CAD build for the part. Positions are in the model's coordinates, mm. Face numbers are marked on the shaded views. A direction names the side the tool comes from. Coordinates: 2 decimals unless noted, no trailing zeros. Loops run counter-clockwise (first coordinate to the right, second up) from the corner with the lowest first, then second, coordinate; pieces in that order, holes last. Notation, with made-up numbers: (71, -34) - (123, -34) arc R25 ccw to (123, -2) - close; hole circle Ø2 at (5, -11). An arc over 180 degrees is marked (long way). Put each result on its own line as item: value.
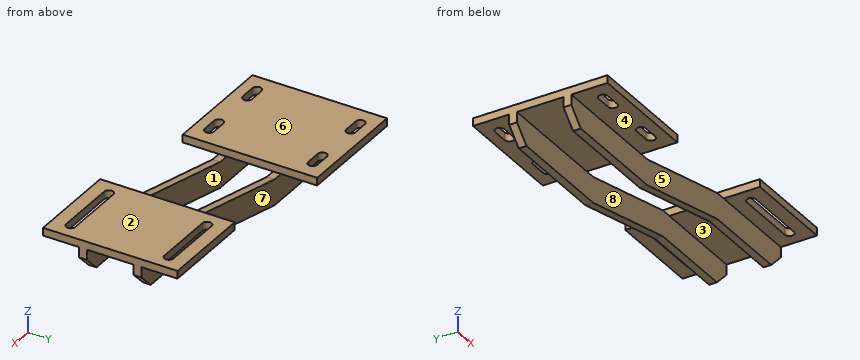
```python
from build123d import *

# Parameters (mm, degrees)
F0_W     = 139.7
F0_H     = 165.1
F1_DEPTH = 9.525
F3_W     = 114.3
F3_H     = 165.1
F4_DEPTH = 9.525
F7_DEPTH = 9.525
F9_SIZE  = 19.05


with BuildPart() as f1:
    # F0 (on Top) → F1 (new body)
    with BuildSketch(Plane.XY):
        Rectangle(F0_W, F0_H)
        with BuildLine():
            ThreePointArc((-47.625, -69.088), (-53.213, -63.5), (-47.625, -57.912))
            Line((-47.625, -57.912), (-28.575, -57.912))
            ThreePointArc((-28.575, -57.912), (-22.987, -63.5), (-28.575, -69.088))
            Line((-28.575, -69.088), (-47.625, -69.088))
        make_face(mode=Mode.SUBTRACT)
        with BuildLine():
            Line((28.575, -57.912), (47.625, -57.912))
            ThreePointArc((47.625, -57.912), (53.213, -63.5), (47.625, -69.088))
            Line((47.625, -69.088), (28.575, -69.088))
            ThreePointArc((28.575, -69.088), (22.987, -63.5), (28.575, -57.912))
        make_face(mode=Mode.SUBTRACT)
        with BuildLine():
            Line((-28.575, 57.912), (-47.625, 57.912))
            ThreePointArc((-47.625, 57.912), (-53.213, 63.5), (-47.625, 69.088))
            Line((-47.625, 69.088), (-28.575, 69.088))
            ThreePointArc((-28.575, 69.088), (-22.987, 63.5), (-28.575, 57.912))
        make_face(mode=Mode.SUBTRACT)
        with BuildLine():
            ThreePointArc((47.625, 69.088), (53.213, 63.5), (47.625, 57.912))
            Line((47.625, 57.912), (28.575, 57.912))
            ThreePointArc((28.575, 57.912), (22.987, 63.5), (28.575, 69.088))
            Line((28.575, 69.088), (47.625, 69.088))
        make_face(mode=Mode.SUBTRACT)
    extrude(amount=-F1_DEPTH)



with BuildPart() as f4:
    # F3 (on offset) → F4 (new body)
    with BuildSketch(Plane.XY.offset(31.75)):
        with Locations((292.1, 0)):
            Rectangle(F3_W, F3_H)
        with BuildLine():
            ThreePointArc((254, -65.913), (248.412, -60.325), (254, -54.737))
            Line((254, -54.737), (330.2, -54.737))
            ThreePointArc((330.2, -54.737), (335.788, -60.325), (330.2, -65.913))
            Line((330.2, -65.913), (254, -65.913))
        make_face(mode=Mode.SUBTRACT)
        with BuildLine():
            Line((330.2, 54.737), (254, 54.737))
            ThreePointArc((254, 54.737), (248.412, 60.325), (254, 65.913))
            Line((254, 65.913), (330.2, 65.913))
            ThreePointArc((330.2, 65.913), (335.788, 60.325), (330.2, 54.737))
        make_face(mode=Mode.SUBTRACT)
    extrude(amount=-F4_DEPTH)


with BuildPart() as f1_1:
    add(f1.part)

    add(f4.part)  # F7 merges F4
    # F6 (on offset) → F7 (join)
    with BuildSketch(Plane.XZ.offset(38.1)):
        Polygon((69.85, -9.525), (-69.85, -9.525), (-69.85, -41.275), (82.55, -41.275), (222.25, -9.525), (349.25, -9.525), (349.25, 22.225), (234.95, 22.225), (222.25, 22.225), (82.55, -9.525), align=None)
    extrude(amount=-F7_DEPTH)

    # F8: F1 across plane


with BuildPart() as f1_2:
    add(f1_1.part)
    add(f1_1.part.mirror(Plane.XZ))

    # F9
    f9_edges = [f1_2.edges().sort_by_distance(p)[0] for p in [
        (-69.85, -33.3375, -41.275),
        (-69.85, 33.3375, -41.275),
        (349.25, -33.3375, -9.525),
        (349.25, 33.3375, -9.525),
    ]]
    chamfer(f9_edges, length=F9_SIZE)


solid = f1_2.part
```
Q1. Wall check: L1, parallel to X at y = 65, z = -6.5; L2, parallel to Y at x = 275, z = 9.5 (3 decimals); L3, parallel to Z at x = 268, y = -41 (3 decimals). Give the ranges that are in metal, low to high. Write a range as from..to.
Determined:
L1: -69.85..-53.01, -23.19..23.19, 53.01..69.85
L2: -38.1..-28.575, 28.575..38.1
L3: 22.225..31.75
Q2. Slice it at A-A, the plane y = -3. Give the cut face in (x, z) (3 decimals).
Determined:
outline: (-69.85, -9.525) - (69.85, -9.525) - (69.85, 0) - (-69.85, 0) - close; (234.95, 22.225) - (349.25, 22.225) - (349.25, 31.75) - (234.95, 31.75) - close
Q3. Pin check, flat tips, straight feed: pin 1 Ø13.5 at (x, y) = (266, 63) entering from -Z (3 decimals); pin 2 Ø10 at (x, z) = (205, -23.5) entering from -Y; pin 3 Ø19 at (x, z) = (221, 0) entering from -Y; pin 4 Ø5 at (x, y) = (260.5, -34.5) entering from -Z (3 decimals). Stop position of each tip, or through.
Determined:
pin 1: z = 22.225
pin 2: through
pin 3: y = -38.1
pin 4: z = -9.525
Q4. Tool access for the marked faces 1, 2, 3 and 4: list every direction of +Z, -Z, +X, -X, +Y, -Y with a clear straight run to the whole face (end or side of a thin tool).
Determined:
face 1: -Z, +X
face 2: +Z, +X, -X, +Y, -Y
face 3: -Z, +X, -X
face 4: -Z, +X, -X, -Y
Q5. Slice it at B-B, the plane x = 188. Give the cut face in (y, z) (3 decimals).
Determined:
outline: (-38.1, -17.309) - (-28.575, -17.309) - (-28.575, 14.441) - (-38.1, 14.441) - close; (28.575, -17.309) - (38.1, -17.309) - (38.1, 14.441) - (28.575, 14.441) - close
Q6. Mould opens along Y. For the marked faces 5, 6, 7 and 8 say: +Y half, -Y half, draft (parallel to the pull), parting line (faces both ways), or undercut.
Determined:
face 5: -Y half
face 6: draft
face 7: +Y half
face 8: undercut
